```python
from build123d import *

# Parameters (mm, degrees)
SKETCH1_W           = 3
SKETCH1_H           = 64
SKETCH1_H_2         = 3
SKETCH1_W_2         = 14
BOSS_EXTRUDE1_DEPTH = 50
SKETCH2_W           = 20
SKETCH2_H           = 70
SKETCH2_W_2         = 14
SKETCH2_H_2         = 64
BOSS_EXTRUDE2_DEPTH = 406.293714059


with BuildPart() as part:
    # Sketch1 → Boss-Extrude1 (new body)
    with BuildSketch(Plane.XY):
        with Locations((1.5, 35)):
            Rectangle(SKETCH1_W, SKETCH1_H)
        with Locations((1.5, 68.5)):
            Rectangle(SKETCH1_W, SKETCH1_H_2)
        with Locations((10, 68.5)):
            Rectangle(SKETCH1_W_2, SKETCH1_H_2)
        with Locations((18.5, 68.5)):
            Rectangle(SKETCH1_W, SKETCH1_H_2)
        with Locations((18.5, 35)):
            Rectangle(SKETCH1_W, SKETCH1_H)
        with Locations((10, 1.5)):
            Rectangle(SKETCH1_W_2, SKETCH1_H_2)
        with Locations((1.5, 1.5)):
            Rectangle(SKETCH1_W, SKETCH1_H_2)
        with Locations((18.5, 1.5)):
            Rectangle(SKETCH1_W, SKETCH1_H_2)
    extrude(amount=-BOSS_EXTRUDE1_DEPTH)

    # Sketch2 → Boss-Extrude2 (add)
    with BuildSketch(Plane.XY):
        with Locations((10, 35)):
            Rectangle(SKETCH2_W, SKETCH2_H)
        with Locations((10, 35)):
            Rectangle(SKETCH2_W_2, SKETCH2_H_2, mode=Mode.SUBTRACT)
    extrude(amount=BOSS_EXTRUDE2_DEPTH)


solid = part.part
```
CAD build for the part. Positions are in the model's coordinates, mm. A direction names the side the tool comes from. Round coordinates to 2 decimals unless told otherwise and drop trailing zeros. Write each loop counter-clockwise with the first axis right and the second up, starting at its lowest first coordinate (ties: lowest second). Pieces come first, ordered by that corner, then holes. Notation, with made-up numbers: (24, 23.5) - (44, 23.5) arc R19 cw to (44, 56.5) - close; hole circle Ø6 at (49, -29). An arc over 180 degrees is marked (long way). Return JSON: item names as keys, results as strings. Group by question number.
Item 1: Band-saw the part on C-C on x = 11.5. List the corners of the cut face in (y, z), plus the area to 3 significant figures.
Item 2: 3-axis set-ups, long thin cutter, end or side, ignore diameter. For faces 1 (the face through (3, 35, 175)), 2 (the face through (0, 35, 175)): which of +Z, -Z, +X, -X, +Y, -Y reach the whole face in a straight line?
Item 3: Band-saw the part on A-A on y = 59. List the corners of the cut face in (x, z), plus the area to 3 significant figures.
Item 4: Band-saw the part on B-B on z = 43. List the corners of the cut face in (x, y).
Item 5: Probe probe 1 along Y at (x, z) = (15.5, 48); probe 2 along X at (y, z) = (44, 219.5). List the from-to ranges inside material, lowest first.
Resolved:
{
 "1": {"outline": "(0, -50) - (3, -50) - (3, 406.29) - (0, 406.29) - close; (67, -50) - (70, -50) - (70, 406.29) - (67, 406.29) - close", "area": "2,740 mm²"},
 "2": {"face 1": "+Z, -Z", "face 2": "+Z, -Z, -X, +Y, -Y"},
 "3": {"outline": "(0, -50) - (3, -50) - (3, 406.29) - (0, 406.29) - close; (17, -50) - (20, -50) - (20, 406.29) - (17, 406.29) - close", "area": "2,740 mm²"},
 "4": {"outline": "(0, 0) - (20, 0) - (20, 70) - (0, 70) - close; hole (3, 3) - (17, 3) - (17, 67) - (3, 67) - close"},
 "5": {"probe 1": "y = 0 to 3, 67 to 70", "probe 2": "x = 0 to 3, 17 to 20"}
}
